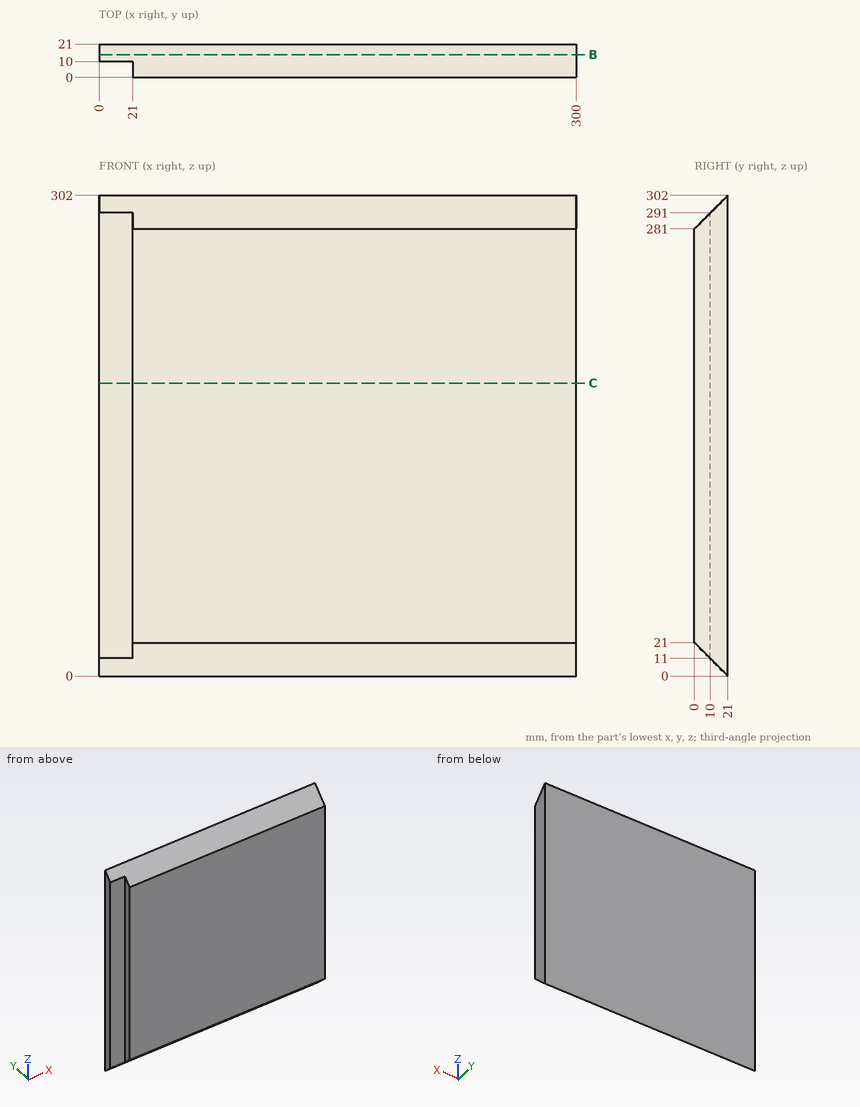
Geometry check sheet. Reference: drawing and pictorial views, mm from the part's lowest x, y, z. Give positions to 0.01 mm unless a question says otherwise; leave off trailing zeros. Write each loop counter-clockwise with the first axis right and the second up, starting at its lowest first coordinate (ties: lowest second). Pieces come first, ordered by that corner, then holes. Notation, with made-up numbers: (8, 83) - (19, 83) arc R11 ccw to (19, 101) - close; hole circle Ø7 at (52, 4). An arc over 180 degrees is marked (long way). Put each result on its own line as item: value.
Q1. Depth check by flat-ended pin: P1, Ø1, axis at x = 263.5, y = 7, coming from the +Z side; P2, Ø8, axis at x = 264.5, y = 5.5, coming from the +Z side; P3, Ø8, axis at y = 4, z = 117.5, coming from the -X side. Enter the tip coordinate at first touch or a pass-through.
Result:
P1: z = 288.5
P2: z = 290.5
P3: x = 21
Q2. Section check B-B on y = 14.25. Record the cut outline in (x, z).
Result:
outline: (0, 6.75) - (300, 6.75) - (300, 295.25) - (0, 295.25) - close
Q3. Section check C-C on z = 184. Record the cut outline in (x, y), and give its area (3 significant figures).
Result:
outline: (0, 10) - (21, 10) - (21, 0) - (300, 0) - (300, 21) - (0, 21) - close
area: 6,090 mm2
Q4. Scan lines: probe 1 along X at (y, z) = (6.75, 200.5); probe 2 along Z at (x, y) = (288.5, 10); probe 3 along Y at (x, z) = (12, 158). Record each from-to range of solid material in increasing order. Write a range as from..to.
Result:
probe 1: 21..300
probe 2: 11..291
probe 3: 10..21
